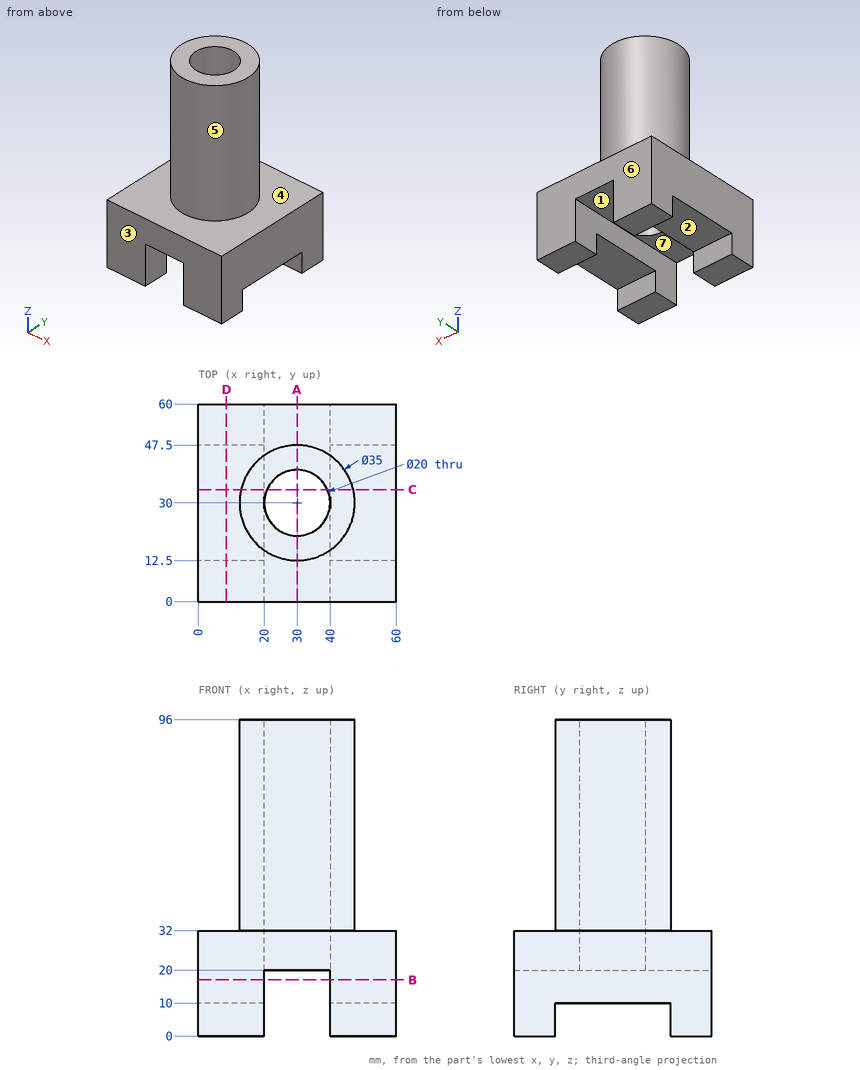
Geometry check sheet. Reference: drawing and pictorial views, mm from the part's lowest x, y, z. A direction names the side the tool comes from. Round coordinates to 2 decimals unless told otherwise and drop trailing zeros. Order: outer loops, then holes, each group sorted by start corner. A loop starts at its lowest first (then second) coordinate and runs counter-clockwise, first axis right, second up.
Q1. Cross-section at C-C, the plane y = 34. Enter the section's corners in (x, z).
Filled sheet:
outline: (0, 10) - (20, 10) - (20, 20) - (20.83, 20) - (20.83, 96) - (12.96, 96) - (12.96, 32) - (0, 32) - close; (39.17, 20) - (40, 20) - (40, 10) - (60, 10) - (60, 32) - (47.04, 32) - (47.04, 96) - (39.17, 96) - close
Q2. Draft check along X on the marked faces 5, 6 and 7. Enter one of: pulls with the +X half, pulls with the -X half, needs draft (parallel to the pull), parting line crosses it, or undercut.
Filled sheet:
face 5: parting line crosses it
face 6: needs draft
face 7: undercut
Q3. Set-up check for the marked faces 1, 2, 3 and 4: record each of +Z, -Z, +X, -X, +Y, -Y from which the full face is reachable in a straight line by a thin tool's end or side.
Filled sheet:
face 1: -Z, +Y, -Y
face 2: -Z, +X, -X
face 3: +Z, -Z, +X, -X, -Y
face 4: +Z
Q4. Depth check by flat-ended pin: P1, Ø3, axis at x = 33.5, y = 47.5, coming from the -Z side; P2, Ø5, axis at y = 38, z = 79, coming from the +X side; P3, Ø1.5, axis at x = 19.5, y = 10.5, coming from the +Z side; P4, Ø1.5, axis at x = 8, z = 33.5, coming from the -Y side. Enter the tip coordinate at first touch or a pass-through.
Filled sheet:
P1: stops at z = 20
P2: stops at x = 46.61
P3: stops at z = 32
P4: passes through
Q5. Cross-section at A-A, the plane x = 30. Enter the section's corners in (y, z), plus the area to 3 significant figures.
Filled sheet:
outline: (0, 20) - (20, 20) - (20, 96) - (12.5, 96) - (12.5, 32) - (0, 32) - close; (40, 20) - (60, 20) - (60, 32) - (47.5, 32) - (47.5, 96) - (40, 96) - close
area: 1,440 mm2
Q6. Scan lines: L1, parallel to X at y = 19, z = 19.5; L2, parallel to Y at x = 30, z = 43; L3, parallel to Z at x = 22, y = 44.5. Record each from-to range of solid material in increasing order.
Filled sheet:
L1: x = 0 to 20, 40 to 60
L2: y = 12.5 to 20, 40 to 47.5
L3: z = 20 to 96
Q7. Cross-section at B-B, the plane z = 17. Enter the section's corners in (x, y).
Filled sheet:
outline: (0, 0) - (20, 0) - (20, 60) - (0, 60) - close; (40, 0) - (60, 0) - (60, 60) - (40, 60) - close
Q8. Cross-section at D-D, the plane x = 8.5. Enter the section's corners in (y, z), plus the area to 3 significant figures.
Filled sheet:
outline: (0, 0) - (12.5, 0) - (12.5, 10) - (47.5, 10) - (47.5, 0) - (60, 0) - (60, 32) - (0, 32) - close
area: 1,570 mm2
